Part model, mm, in its own coordinate system. A direction names the side the tool comes from. Coordinates: 2 decimals unless noted, no trailing zeros. Write each loop counter-clockwise with the first axis right and the second up, starting at its lowest first coordinate (ties: lowest second). Pieces come first, ordered by that corner, then holes. Notation, with made-up numbers: (-29, 78.25) - (-8, 78.25) arc R26 cw to (-8, 108.25) - close; hole circle Ø9 at (9.25, 55). An arc over 180 degrees is marked (long way). Write each question's results on one line, items separated by ' | '.
from build123d import *

# Parameters (mm, degrees)
SKETCH1_R                = 24
BOSS_EXTRUDE4_DEPTH      = 77.8
BOSS_EXTRUDE4_DEPTH_BACK = 0.01
SKETCH6_R                = 30.26307147
CUT_EXTRUDE1_DEPTH       = 8
SKETCH9_R                = 30.265
CUT_EXTRUDE2_DEPTH       = 8


with BuildPart() as part:
    # Sketch1 → Boss-Extrude4 (new body, two sides)
    with BuildSketch(Plane.XY) as boss_extrude4_sk:
        with BuildLine():
            Line((-240.6, 12.003445454), (78.3, 12.003445454))
            ThreePointArc((78.3, 12.003445454), (115.2, -24.896554546), (78.3, -61.796554546))
            Line((78.3, -61.796554546), (-240.6, -61.796554546))
            ThreePointArc((-240.6, -61.796554546), (-277.5, -24.896554546), (-240.6, 12.003445454))
        make_face()
        with Locations((-240.6, -24.896554546)):
            Circle(SKETCH1_R, mode=Mode.SUBTRACT)
        with Locations((-160.9, -24.896554546)):
            Circle(SKETCH1_R, mode=Mode.SUBTRACT)
        with Locations((-81.2, -24.896554546)):
            Circle(SKETCH1_R, mode=Mode.SUBTRACT)
        with Locations((-1.5, -24.896554546)):
            Circle(SKETCH1_R, mode=Mode.SUBTRACT)
        with Locations((78.3, -24.896554546)):
            Circle(SKETCH1_R, mode=Mode.SUBTRACT)
    extrude(amount=BOSS_EXTRUDE4_DEPTH)
    extrude(boss_extrude4_sk.sketch, amount=-BOSS_EXTRUDE4_DEPTH_BACK)

    # Sketch6 → Cut-Extrude1 (cut)
    with BuildSketch(Plane.XY.offset(77.8)):
        with Locations((-240.6, -24.896554546)):
            Circle(SKETCH6_R)
        with Locations((-160.9, -24.896554546)):
            Circle(SKETCH6_R)
        with Locations((-81.2, -24.896554546)):
            Circle(SKETCH6_R)
        with Locations((-1.5, -24.896554546)):
            Circle(SKETCH6_R)
        with Locations((78.2, -24.896554546)):
            Circle(SKETCH6_R)
    extrude(amount=-CUT_EXTRUDE1_DEPTH, mode=Mode.SUBTRACT)

    # Sketch9 → Cut-Extrude2 (cut)
    with BuildSketch(Plane(origin=(0, 0, -0.01), x_dir=(-1, 0, 0), z_dir=(0, 0, -1))):
        with Locations((-78.3, -24.896554546)):
            Circle(SKETCH9_R)
        with Locations((1.4, -24.896554546)):
            Circle(SKETCH9_R)
        with Locations((81.1, -24.896554546)):
            Circle(SKETCH9_R)
        with Locations((160.8, -24.896554546)):
            Circle(SKETCH9_R)
        with Locations((240.5, -24.896554546)):
            Circle(SKETCH9_R)
    extrude(amount=-CUT_EXTRUDE2_DEPTH, mode=Mode.SUBTRACT)


solid = part.part
(1) Two-plate mould, pull along Y, no slides. Class faces 4 (the flat face through (-63, -9, 7.99)), 5 (the flat face through (17, -9, 7.99)), 6 (the flat face through (-78, -57, -0.01)), 7 (the flat face through (-79, -61.797, 39)): released by +Y, released by -Y, zero draft, split by the parting line, or undercut.
Return value:
face 4: undercut | face 5: undercut | face 6: zero draft | face 7: released by -Y
(2) Saw through at B-B on z = 22. Write the cut outline in (x, y), then the cut area to 3 significant figures.
Return value:
outline: (-240.6, -61.8) - (78.3, -61.8) arc R36.9 ccw to (78.3, 12) - (-240.6, 12) arc R36.9 ccw to start; hole circle Ø48 at (-240.6, -24.9); hole circle Ø48 at (-160.9, -24.9); hole circle Ø48 at (-81.2, -24.9); hole circle Ø48 at (-1.5, -24.9); hole circle Ø48 at (78.3, -24.9) | area: 18,800 mm^2
(3) Wall check: line 1 (Y direction, x = 78.3, z = 5.5); line 2 (Y direction, x = -240, z = 23); line 3 (X direction, y = -20, z = 10). Give the ranges that are in metal, low to high. Write a range as from..to.
Return value:
line 1: y = -61.8..-55.16, 5.37..12 | line 2: y = -61.8..-48.89, -0.9..12 | line 3: x = -277.17..-264.1, -217.1..-184.4, -137.4..-104.7, -57.7..-25, 22..54.8, 101.8..114.87
(4) Saw through at A-A on x = -1.4. Write the cut outline in (y, z).
Return value:
outline: (-61.8, -0.01) - (-55.16, -0.01) - (-55.16, 7.99) - (-48.9, 7.99) - (-48.9, 69.8) - (-55.16, 69.8) - (-55.16, 77.8) - (-61.8, 77.8) - close; (-0.9, 7.99) - (5.37, 7.99) - (5.37, -0.01) - (12, -0.01) - (12, 77.8) - (5.37, 77.8) - (5.37, 69.8) - (-0.9, 69.8) - close
(5) Saw through at D-D on y = -8.5. Count the separate pieces of the cut face and the enclosed holes in it, then the cut area to 3 significant figures.
Return value:
separate pieces: 6 | enclosed holes: 0 | area: 15,100 mm^2
(6) 3-axis set-ups, long thin cutter, end or side, ignore diameter. For faces 1 (the cylindrical face through (-8.06, -54.44, 73.86)), 2 (the flat face through (-170, -2, 7.99)), 3 (the cylindrical face through (-105.177, -23.841, 39.328)): which of +Z, -Z, +X, -X, +Y, -Y reach the whole face in a straight line?
Return value:
face 1: +Z | face 2: -Z | face 3: +Z, -Z
(7) Flat gauge pins, fed straight in: P1, Ø1, axis at y = -30.5, z = 62, coming from the +X side; P2, Ø8, axis at y = -38.5, z = 55, coming from the +X side; P3, Ø18, axis at x = -236.5, y = -36, coming from the +Z side; P4, Ø1, axis at x = -56.5, y = -29, coming from the +Z side. Where does each tip first touch, or does it go through?
Return value:
P1: stops at x = 114.85 | P2: stops at x = 113.93 | P3: passes through | P4: stops at z = 69.8
